Input: part model. Units: mm. Frame: model coordinates. A direction names the side the tool comes from. Coordinates: 2 decimals unless noted, no trailing zeros. Write each loop counter-clockwise with the first axis right and the second up, starting at its lowest first coordinate (ties: lowest second). Pieces come first, ordered by that corner, then holes. Notation, with made-up numbers: M 3.5,19 L 24.5,19 A23 cw 24.5,30 Z; hole C 8,-40 d6. An arc over 180 degrees is marked long. Use one line per item in the form item = value.
from build123d import *

# Parameters (mm, degrees)
CYLINDER002_R     = 31.5
CYLINDER002_DEPTH = 5
CYLINDER003_R     = 43.5
CYLINDER003_DEPTH = 5
CYLINDER_R        = 38.5
CYLINDER_DEPTH    = 60
CYLINDER001_R     = 43.5
CYLINDER001_DEPTH = 60


with BuildPart() as interior_cono:
    # Cone → Cone (revolve)
    with BuildSketch(Plane.XZ):
        Polygon((0, 0), (27.5, 0), (31.25, 64), (0, 64), align=None)
    revolve(axis=Axis((0, 0, 0), (0, 0, 1)))


with BuildPart() as cono_inferior:
    # Cone001 → Cone001 (revolve)
    with BuildSketch(Plane.XZ):
        Polygon((0, 0), (32.5, 0), (36.25, 64), (0, 64), align=None)
    revolve(axis=Axis((0, 0, 0), (0, 0, 1)))

    # Cut001: cut Interior_cono
    add(interior_cono.part, mode=Mode.SUBTRACT)


with BuildPart() as obj1:
    # Cylinder002 → Cylinder002 (new body)
    with BuildSketch(Plane.XY):
        Circle(CYLINDER002_R)
    extrude(amount=CYLINDER002_DEPTH)


with BuildPart() as obj2:
    # Cylinder003 → Cylinder003 (new body)
    with BuildSketch(Plane.XY):
        Circle(CYLINDER003_R)
    extrude(amount=CYLINDER003_DEPTH)

    # Cut002: cut obj1
    add(obj1.part, mode=Mode.SUBTRACT)


with BuildPart() as obj2_1:
    # Cut002 placement: moved
    add(obj2.part.moved(Location((0, 0, 64))))


with BuildPart() as obj3:
    # Cylinder → Cylinder (new body)
    with BuildSketch(Plane.XY):
        Circle(CYLINDER_R)
    extrude(amount=CYLINDER_DEPTH)


with BuildPart() as parte:
    # Cylinder001 → Cylinder001 (new body)
    with BuildSketch(Plane.XY):
        Circle(CYLINDER001_R)
    extrude(amount=CYLINDER001_DEPTH)

    # Cut: cut obj3
    add(obj3.part, mode=Mode.SUBTRACT)


with BuildPart() as parte_1:
    # Cut placement: moved
    add(parte.part.moved(Location((0, 0, 69))))

    # Fusion: union Cono_inferior, obj2
    add(cono_inferior.part)
    add(obj2_1.part)


solid = parte_1.part
(1) Set-up query: faces 1 (the cylindrical face through (-30.55, -23.43, 98.58)), 2 (the cylindrical face through (-5.66, 43.13, 96.04)). Return all of +Z, -Z, +X, -X, +Y, -Y with unobstructed straight access to the full face (end or side cutting, diameter ignored); none if empty.
Computed:
face_1 = +Z
face_2 = +Z, -Z
(2) First-contact query: pin 1 Ø12 at (y, z) = (16, 22) entering from -X; pin 2 Ø1 at (x, z) = (-24.5, 70.5) entering from -Y; pin 3 Ø8 at (y, z) = (13.5, 101) entering from -X; pin 4 Ø12 at (x, y) = (-16.5, 31) entering from +Z. Flat tips, straight axial feed; report the tip coordinate or a pass-through.
Computed:
pin_1 = -32.31
pin_2 = -36.28
pin_3 = -42.45
pin_4 = 129
(3) Line query: probe 1 along Y at (x, z) = (0, 91); probe 2 along Y at (x, z) = (0, 65); probe 3 along Z at (x, y) = (38.5, -7.5). Output: solid intervals per line, ascending.
Computed:
probe_1 = -43.5 to -38.5, 38.5 to 43.5
probe_2 = -43.5 to -31.5, 31.5 to 43.5
probe_3 = 64 to 129
(4) Section query A-A on y = 0. Return the cut outline in (x, z), plus the area to 3 significant figures.
Computed:
outline = M -43.5,64 L -36.25,64 L -32.5,0 L -27.5,0 L -31.25,64 L -31.5,64 L -31.5,69 L -38.5,69 L -38.5,129 L -43.5,129 Z; M 27.5,0 L 32.5,0 L 36.25,64 L 43.5,64 L 43.5,129 L 38.5,129 L 38.5,69 L 31.5,69 L 31.5,64 L 31.25,64 Z
area = 1,360 mm^2
(5) Section query D-D on z = 22.5. Return the cut outline in (x, y).
Computed:
outline = C 0,0 d67.64; hole C 0,0 d57.64
(6) Pull-direction query (Y, two-part tool) for faces 3 (the flat face through (-32, 0, 69)), 4 (the conical face through (-27.3, -20.93, 32.45)), 5 (the flat face through (-10, 36, 64)); classes: pulls with the +Y half, pulls with the -Y half, needs draft (parallel to the pull), parting line crosses it, or undercut.
Computed:
face_3 = undercut
face_4 = parting line crosses it
face_5 = needs draft
(7) Section query C-C on z = 101.5. Return the cut outline in (x, y).
Computed:
outline = C 0,0 d87; hole C 0,0 d77
